from build123d import *

# Parameters (mm, degrees)
SKETCH1_R           = 2.5
BOSS_EXTRUDE3_DEPTH = 1.5
FILLET1_R           = 2.5


with BuildPart() as part:
    # Sketch1 → Boss-Extrude3 (new body)
    with BuildSketch(Plane(origin=(0, 0, 0), x_dir=(0, 0, -1), z_dir=(1, 0, 0))):
        with BuildLine():
            Line((-34.72862652, 4.35), (-33.15, 4.35))
            Line((-33.15, 4.35), (-33.15, -4.35))
            Line((-33.15, -4.35), (-34.72862652, -4.35))
            ThreePointArc((-34.72862652, -4.35), (-24.748737342, -24.748737342), (-4.35, -34.72862652))
            Line((-4.35, -34.72862652), (-4.35, -33.15))
            Line((-4.35, -33.15), (4.35, -33.15))
            Line((4.35, -33.15), (4.35, -34.72862652))
            ThreePointArc((4.35, -34.72862652), (24.748737342, -24.748737342), (34.72862652, -4.35))
            Line((34.72862652, -4.35), (33.15, -4.35))
            Line((33.15, -4.35), (33.15, 4.35))
            Line((33.15, 4.35), (34.72862652, 4.35))
            ThreePointArc((34.72862652, 4.35), (24.748737342, 24.748737342), (4.35, 34.72862652))
            Line((4.35, 34.72862652), (4.35, 33.15))
            Line((4.35, 33.15), (-4.35, 33.15))
            Line((-4.35, 33.15), (-4.35, 34.72862652))
            ThreePointArc((-4.35, 34.72862652), (-24.748737342, 24.748737342), (-34.72862652, 4.35))
        make_face()
        Circle(SKETCH1_R, mode=Mode.SUBTRACT)
        with BuildLine():
            Line((9.270248109, 3.75), (27.243118397, 3.75))
            ThreePointArc((27.243118397, 3.75), (19.17641557, 19.71078603), (3, 27.335873866))
            Line((3, 27.335873866), (3, 9.539392014))
            ThreePointArc((3, 9.539392014), (6.783731432, 7.347175502), (9.270248109, 3.75))
        make_face(mode=Mode.SUBTRACT)
        with BuildLine():
            Line((-3, 9.539392014), (-3, 27.335873866))
            ThreePointArc((-3, 27.335873866), (-19.709993452, 19.177230199), (-27.407799985, 2.25))
            Line((-27.407799985, 2.25), (-9.743587635, 2.25))
            ThreePointArc((-9.743587635, 2.25), (-7.340542585, 6.790908228), (-3, 9.539392014))
        make_face(mode=Mode.SUBTRACT)
        with BuildLine():
            Line((9.743587635, -2.25), (27.407799985, -2.25))
            ThreePointArc((27.407799985, -2.25), (20.230473673, -18.627343744), (4.5, -27.129319933))
            Line((4.5, -27.129319933), (4.5, -8.93028555))
            ThreePointArc((4.5, -8.93028555), (7.866161766, -6.174422974), (9.743587635, -2.25))
        make_face(mode=Mode.SUBTRACT)
        with BuildLine():
            Line((-1.5, -9.886859967), (-1.5, -27.459060435))
            ThreePointArc((-1.5, -27.459060435), (-18.629857769, -20.22815858), (-27.243118397, -3.75))
            Line((-27.243118397, -3.75), (-9.270248109, -3.75))
            ThreePointArc((-9.270248109, -3.75), (-6.197969316, -7.847622338), (-1.5, -9.886859967))
        make_face(mode=Mode.SUBTRACT)
    extrude(amount=BOSS_EXTRUDE3_DEPTH)

    # Fillet1
    fillet1_edges = [part.edges().sort_by_distance(p)[0] for p in [
        (0.75, -9.886859967, 1.5),
        (0.75, -3.75, 9.270248109),
        (0.75, -3.75, 27.243118397),
        (0.75, -27.459060435, 1.5),
        (0.75, 27.335873866, 3),
        (0.75, 2.25, 27.407799985),
        (0.75, 2.25, 9.743587635),
        (0.75, 9.539392014, 3),
        (0.75, 3.75, -27.243118397),
        (0.75, 27.335873866, -3),
        (0.75, 9.539392014, -3),
        (0.75, 3.75, -9.270248109),
        (0.75, -2.25, -9.743587635),
        (0.75, -8.93028555, -4.5),
        (0.75, -27.129319933, -4.5),
        (0.75, -2.25, -27.407799985),
    ]]
    fillet(fillet1_edges, radius=FILLET1_R)


solid = part.part
Work out the finished part from the listing and answer in its coordinate system (mm). A direction names the side the tool comes from. Give positions to 0.01 mm unless a question says otherwise; leave off trailing zeros. Loops run counter-clockwise (first coordinate to the right, second up) from the corner with the lowest first, then second, coordinate; pieces in that order, holes last. Notation, with made-up numbers: (47, 67.25) -> (69, 67.25) arc R22 cw to (69, 85.25) -> close; hole circle Ø5 at (52, -32.75). An arc over 180 degrees is marked (long way). Use a Markdown table: item, result. Add a question column.
1. Section D-D on y = 23.5 is taken. Determine the outline of the cut face in (x, z), and give its area (3 significant figures).
2. Find the intervals of material crossed by probe 1 along Z at (x, y) = (1, -20.5); probe 2 along Y at (x, z) = (0.4, 21.5); probe 3 along Y at (x, z) = (1, 0), in increasing order.
3. Section C-C on z = 16 is taken. Determine the outline of the cut face in (x, y), and give its area (3 significant figures).
4. For faces 1 (the flat face through (1, 4.35, -34)), 2 (the flat face through (1, 18, 3)), 3 (the flat face through (1, 0, 33.15)), determine the directions among +Z, -Z, +X, -X, +Y, -Y from which every point of the face is accessible in a straight line to the end or side of a thin tool.
5. A flat-ended cylindrical pin translates along its axis: pin 1 Ø0.8 at (x, z) = (1, 16) entering from -Y. Find the tip coordinate at first contact, or state that the pin passes through.
6. Determine the mould class of faces 4 (the cylindrical face through (0.76, 9.886, -3.389)), 5 (the flat face through (1.5, 0, -7)), 6 (the cylindrical face through (0.74, 24.977, 24.519)) for opening direction Z: released by +Z, released by -Z, zero draft, split by the parting line, or undercut.
7. Section A-A on z = 0 is taken. Determine the outline of the cut face in (x, y), and give its area (4 significant figures).
Results below:
| question | item | result |
|---|---|---|
| 1 | outline | (0, -25.94) -> (1.5, -25.94) -> (1.5, -14.28) -> (0, -14.28) -> close; (0, -3) -> (1.5, -3) -> (1.5, 3) -> (0, 3) -> close; (0, 14.28) -> (1.5, 14.28) -> (1.5, 25.94) -> (0, 25.94) -> close |
| 1 | area | 44.0 mm^2 |
| 2 | probe 1 | z = -28.37 to -18.33, -4.5 to 1.5, 18.33 to 28.37 |
| 2 | probe 2 | y = -27.62 to -17.15, -3.75 to 2.25, 17.15 to 27.62 |
| 2 | probe 3 | y = -33.15 to -2.5, 2.5 to 33.15 |
| 3 | outline | (0, -31.13) -> (1.5, -31.13) -> (1.5, -22.37) -> (0, -22.37) -> close; (0, -3.75) -> (1.5, -3.75) -> (1.5, 2.25) -> (0, 2.25) -> close; (0, 22.37) -> (1.5, 22.37) -> (1.5, 31.13) -> (0, 31.13) -> close |
| 3 | area | 35.3 mm^2 |
| 4 | face 1 | -Z, +X, -X |
| 4 | face 2 | +X, -X |
| 4 | face 3 | +Z, +X, -X |
| 5 | pin 1 | stops at y = -31.33 |
| 6 | face 4 | undercut |
| 6 | face 5 | zero draft |
| 6 | face 6 | released by +Z |
| 7 | outline | (0, -33.15) -> (1.5, -33.15) -> (1.5, -2.5) -> (0, -2.5) -> close; (0, 2.5) -> (1.5, 2.5) -> (1.5, 33.15) -> (0, 33.15) -> close |
| 7 | area | 91.95 mm^2 |
